Read the model definition and answer for the solid it produces. Units are mm, in the model's axes. Face numbers are marked on the shaded views. A direction names the side the tool comes from. Coordinates: 2 decimals unless noted, no trailing zeros. Loops run counter-clockwise (first coordinate to the right, second up) from the corner with the lowest first, then second, coordinate; pieces in that order, holes last. Notation, with made-up numbers: (-35.5, 32.25) - (-18.5, 32.25) arc R18 ccw to (-18.5, 53.25) - close; hole circle Ø6 at (0.5, 83). An arc over 180 degrees is marked (long way). Use one line per item in the form item = value.
Autodesk Inventor part; units mm, degrees
ref_plane "YZ Plane" through (0, 0, 0) normal (1, 0, 0) x (0, 1, 0)
ref_plane "XZ Plane" through (0, 0, 0) normal (0, 1, 0) x (-1, 0, 0)
ref_plane "XY Plane" through (0, 0, 0) normal (0, 0, 1) x (1, 0, 0)
sketch "Sketch1" plane through (0, 0, 0) normal (0, 1, 0) x (-1, 0, 0)
  circle A0 centre (0, 0) radius 30 construction
  circle A1 centre (0, 0) radius 32.5 construction
  line L0 (0, -30) -> (-81.4496, -30) construction
  circle A2 centre (-81.4496, 0) radius 30 construction
  circle A3 centre (-81.4496, 0) radius 32.5 construction
  line L1 (0, -32.5) -> (-81.4496, -32.5) construction
  line L2 (0, 32.5) -> (-81.4496, 32.5) construction
  line L3 (0, 30) -> (-81.4496, 30) construction
  line L4 (-40.7248, -32.5) -> (-40.7248, 32.5) construction
  line L5 (-40.7248, 30) -> (-40.7248, 14.2852) construction
  line L6 (-81.4496, -30) -> (-81.4496, 30) construction
  line L7 (-40.7248, 14.2852) -> (-40.7248, 16.7852) construction
  arc A4 (0, -30) -> (30, 0) centre (0, 0) ccw
  arc A5 (30, 0) -> (0, 30) centre (0, 0) ccw
  arc A6 (-111.4496, 0) -> (-81.4496, -30) centre (-81.4496, 0) ccw
  arc A7 (-81.4496, 30) -> (-111.4496, 0) centre (-81.4496, 0) ccw
  arc A8 (0, -32.5) -> (32.5, 0) centre (0, 0) ccw
  arc A9 (32.5, 0) -> (0, 32.5) centre (0, 0) ccw
  arc A10 (-81.4496, 32.5) -> (-113.9496, 0) centre (-81.4496, 0) ccw
  arc A11 (-113.9496, 0) -> (-81.4496, -32.5) centre (-81.4496, 0) ccw
  line L8 (0, -30) -> (-81.4496, -30)
  line L9 (0, -32.5) -> (-81.4496, -32.5)
  line L10 (-40.7248, -30) -> (-40.7248, 15) construction
  line L11 (-40.7248, 15) -> (-28.8314, 15) construction
  line L12 (-40.7248, 15) -> (-52.6182, 15) construction
  line L13 (-40.7248, 15) -> (-40.7248, 17.5) construction
  line L14 (-40.7248, 17.5) -> (-27.3861, 17.5)
  line L15 (-40.7248, 17.5) -> (-54.0635, 17.5)
  line L16 (-52.6182, 15) -> (-55.4688, 15) construction
  line L17 (-28.8314, 15) -> (-25.9836, 15) construction
  arc A12 (0, 30) -> (-25.9836, 14.9951) centre (0, 0) ccw
  arc A13 (-55.4688, 15) -> (-81.4496, 30) centre (-81.4496, 0) ccw
  line L18 (-25.9836, 14.9951) -> (-55.4688, 15)
  arc A14 (0, 32.5) -> (-27.3861, 17.5) centre (0, 0) ccw
  arc A15 (-54.0635, 17.5) -> (-81.4496, 32.5) centre (-81.4496, 0) ccw
  circle A16 centre (0, 0) radius 12.5
  line L19 (-81.4496, 0) -> (-81.4496, -4.25) construction
  line L20 (-81.4496, 0) -> (-81.4496, 4.25) construction
  line L21 (-81.4496, 0) -> (-77.1996, 0) construction
  line L22 (-81.4496, 0) -> (-85.6996, 0) construction
  line L23 (-77.1996, 0) -> (-77.1996, -4.25)
  line L24 (-77.1996, -4.25) -> (-85.6996, -4.25)
  line L25 (-85.6996, -4.25) -> (-85.6996, 4.25)
  line L26 (-85.6996, 4.25) -> (-77.1996, 4.25)
  line L27 (-77.1996, 4.25) -> (-77.1996, 0)
  line L28 (-81.4496, -4.25) -> (-81.4496, -5.75) construction
  line L29 (-85.6996, 0) -> (-87.1996, 0) construction
  line L30 (-81.4496, 4.25) -> (-81.4496, 5.75) construction
  line L31 (-77.1996, 0) -> (-75.6996, 0) construction
  line L32 (-77.1996, 4.25) -> (-75.6996, 4.25) construction
  line L33 (-75.6996, 4.25) -> (-75.6996, -3.75)
  line L34 (-75.6996, -3.75) -> (-69.6996, -3.75)
  line L35 (-69.6996, -3.75) -> (-69.6996, 4.25)
  line L36 (-69.6996, 4.25) -> (-75.6996, 4.25)
  line L37 (-87.1996, -4.25) -> (-87.1996, 3.75)
  line L38 (-87.1996, 3.75) -> (-93.1996, 3.75)
  line L39 (-93.1996, 3.75) -> (-93.1996, -4.25)
  line L40 (-93.1996, -4.25) -> (-87.1996, -4.25)
  line L41 (-81.4496, -5.75) -> (-77.4496, -5.75)
  line L42 (-81.4496, -5.75) -> (-85.4496, -5.75)
  line L43 (-85.4496, -5.75) -> (-85.4496, -11.75)
  line L44 (-85.4496, -11.75) -> (-77.4496, -11.75)
  line L45 (-77.4496, -11.75) -> (-77.4496, -5.75)
  line L46 (-81.4496, 5.75) -> (-77.4496, 5.75)
  line L47 (-81.4496, 5.75) -> (-85.4496, 5.75)
  line L48 (-85.4496, 5.75) -> (-85.4496, 11.75)
  line L49 (-85.4496, 11.75) -> (-77.4496, 11.75)
  line L50 (-77.4496, 11.75) -> (-77.4496, 5.75)
  line L51 (0, 0) -> (-16, 0) construction
  line L52 (0, 0) -> (-15, 0) construction
  line L53 (0, 0) -> (-14, 0) construction
  line L54 (0, 12.5) -> (-16, 12.5) construction
  line L55 (0, -12.5) -> (-16, -12.5) construction
  line L56 (-15, 0) -> (-15, 12.5) construction
  line L57 (-15, 0) -> (-15, -12.5) construction
  line L58 (-14, 0) -> (-14, -12.5) construction
  line L59 (-14, 0) -> (-14, 12.5) construction
  line L60 (-16, 12.5) -> (-16, 0) construction
  line L61 (-16, 0) -> (-16, -12.5) construction
  line L62 (-16, -12.5) -> (-16, -8.5) construction
  line L63 (-16, 12.5) -> (-16, 8.5) construction
  line L64 (-14, -12.5) -> (-14, -8.5) construction
  line L65 (-14, 12.5) -> (-14, 8.5) construction
  line L66 (-14, -8.5) -> (-33, -8.5)
  line L67 (-14, 8.5) -> (-14, -8.5)
  line L68 (-14, -12.5) -> (-14, -7.5) construction
  line L69 (-14, 12.5) -> (-14, 7.5) construction
  line L70 (-15, -7.5) -> (-15, 7.5)
  line L71 (-14, 8.5) -> (-33, 8.5)
  line L72 (-33, 7.5) -> (-33, 8.5)
  line L73 (-15, 7.5) -> (-33, 7.5)
  line L74 (-15, -7.5) -> (-33, -7.5)
  line L75 (-33, -7.5) -> (-33, -8.5)
  line L76 (-33, -7.5) -> (-33, 7.5)
  line L77 (0, -12.5) -> (0, -15.5) construction
  line L78 (0, 12.5) -> (0, 15.5) construction
  line L79 (12.5, 0) -> (15.5, 0) construction
  line L80 (15.5, 0) -> (15.5, -15.5)
  line L81 (15.5, -15.5) -> (0, -15.5)
  line L82 (0, 15.5) -> (15.5, 15.5)
  line L83 (15.5, 15.5) -> (15.5, 0)
  line L84 (-33, 0) -> (-36, 0) construction
  line L85 (-36, 0) -> (-36, -15.5)
  line L86 (-36, -15.5) -> (0, -15.5)
  line L87 (15.5, 15.5) -> (-25.6856, 15.5)
  line L88 (-36, 0) -> (-36, 14.9967)
  point P0 (-81.4496, -4.25)
  point P1 (-79.4496, 5.75)
  dimension "d0" = 60
  dimension "d1" = 65
  dimension "d2" = 81.4496
  dimension "d3" = 60
  dimension "d4" = 65
  dimension "d7" = 2.5
  dimension "d10" = 2.5
  dimension "d12" = 25
  dimension "d13" = 81.4496
  dimension "d14" = 2.5
  dimension "d15" = 4.25
  dimension "d16" = 4.25
  dimension "d17" = 4.25
  dimension "d18" = 4.25
  dimension "d21" = 1.5
  dimension "d23" = 8
  dimension "d24" = 6
  dimension "d25" = 50
  dimension "d26" = 45
  dimension "d27" = 25.75
  dimension "d28" = 25.75
  dimension "d29" = 8
  dimension "d30" = 6
  dimension "d32" = 4
  dimension "d33" = 4
  dimension "d34" = 6
  dimension "d35" = 4
  dimension "d36" = 4
  dimension "d37" = 6
  dimension "d38" = 1.5
  dimension "d40" = 1.5
  dimension "d41" = 1.5
  dimension "d42" = 1.5
  dimension "d43" = 8
  dimension "d44" = 16
  dimension "d45" = 15
  dimension "d46" = 14
  dimension "d49" = 4
  dimension "d50" = 4
  dimension "d51" = 19
  dimension "d53" = 5
  dimension "d54" = 5
  dimension "d55" = 19
  dimension "d56" = 18
  dimension "d57" = 18
  dimension "d58" = 15
  dimension "d59" = 3
  dimension "d60" = 3
  dimension "d61" = 3
  dimension "d62" = 3
extrude "Extrusion1" add sketch "Sketch1" against normal blind 35 contours L9 A11 A10 A15 L15 L14 A14 A9 A8
extrude "Extrusion2" add sketch "Sketch1" against normal blind 2.5 contours L87 L82 L83 L80 L81 L86 L85 L88 L18 A12
extrude "Extrusion3" add sketch "Sketch1" against normal blind 4 contours L76 L73 L70 L74
extrude "Extrusion4" add sketch "Sketch1" against normal blind 20 contours L66 L75 L74 L70 L73 L72 L71 L67
extrude "Extrusion5" add sketch "Sketch1" against normal blind 5 contours L8 A6 A7 A13 L18 L88 L85 L86 L81 L80 L83 L82 L87 A12 A5 A4
extrude "Extrusion6" add sketch "Sketch1" against normal blind 1 contours L23 L24 L25 L26 L27
properties part number "controller_v9_d1_3DPrint"
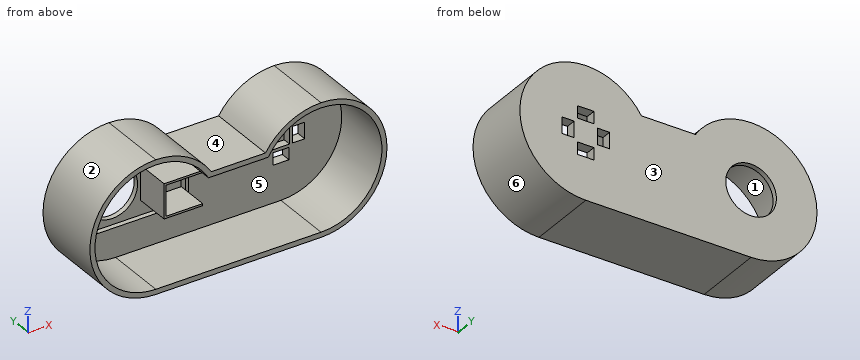
Item 1: The part is cut by section B-B on z = 0. Count the separate pieces of the cut face and the enclosed holes in it, plus the area to 3 significant figures.
Results below:
separate_pieces = 4
enclosed_holes = 0
area = 641 mm²
Item 2: The part is cut by section C-C on x = 104.5. Give the vertices of the cut face in (y, z).
Results below:
outline = (-35, -22.91) - (0, -22.91) - (0, 22.91) - (-35, 22.91) - (-35, 19.2) - (-5, 19.2) - (-5, -19.2) - (-35, -19.2) - close
Item 3: Each of these flat-tipped pins is pushed along its axis until it touches: P1, Ø2, axis at x = 11, y = -3.5, coming from the +Z side; P2, Ø1.2, axis at y = -3.5, z = -3.5, coming from the +X side; P3, Ø5, axis at y = -11.5, z = 20, coming from the +X side. Where does it stop, or does it pass through?
Results below:
P1 = 30.92
P2 = 113.82
P3 = 108.84
Item 4: Which of the six approach directions +Z, -Z, +X, -X, +Y, -Y give full straight-line access (tool end or side, diameter ignored) to the marked faces 4, 5 and 6?
Results below:
face_4 = +Z, +Y, -Y
face_5 = -Y
face_6 = +X, +Y, -Y
Item 5: The part is cut by section D-D on x = 62. Give the vertices of the cut face in (y, z), plus the area to 3 significant figures.
Results below:
outline = (-35, -32.5) - (0, -32.5) - (0, 26.04) - (-35, 26.04) - (-35, 22.84) - (-5, 22.84) - (-5, -30) - (-35, -30) - close
area = 464 mm²
Item 6: For a pull along X with two mould halves and no side action, classify the marked faces 1, 2 and 3 as +X half, -X half, draft (parallel to the pull), parting line (faces both ways), or undercut.
Results below:
face_1 = undercut
face_2 = -X half
face_3 = draft
Item 7: The part is cut by section A-A on y = -30. Give the vertices of the cut face in (x, z).
Results below:
outline = (0, -32.5) - (81.45, -32.5) arc R32.5 ccw to (81.45, 32.5) arc R32.5 ccw to (54.06, 17.5) - (27.39, 17.5) arc R32.5 ccw to (0, 32.5) arc R32.5 ccw to start; hole (0, -30) - (81.45, -30) arc R30 ccw to (81.45, 30) arc R30 ccw to (55.47, 15) - (25.98, 15) arc R30 ccw to (0, 30) arc R30 ccw to start
Item 8: Find the intervals of material crossed by L1, parallel to Z at x = 32, y = -8; L2, parallel to Z at x = 0, y = -1.25; L3, parallel to X at y = -19, z = -7, in increasing order.
Results below:
L1 = -32.5 to -30, -8.5 to -7.5, 7.5 to 8.5, 15 to 17.5
L2 = -32.5 to -12.5, 12.5 to 32.5
L3 = -31.74 to -29.17, 14 to 15, 110.62 to 113.19
